Study the drawing (mm; zero at the part's minimum x, y, z) and answer. Coordinates: 2 decimals unless noted, no trailing zeros. Loops run counter-clockwise (first coordinate to the right, second up) from the corner with the lowest first, then second, coordinate; pieces in that order, holes last. Notation, with made-up numbers: (-40, 60) - (-11, 60) arc R14 ccw to (-11, 79) - close; hole circle Ø8 at (20, 61.5). An arc over 180 degrees is marked (long way). One line per item, written item: value. Start each with the question number.
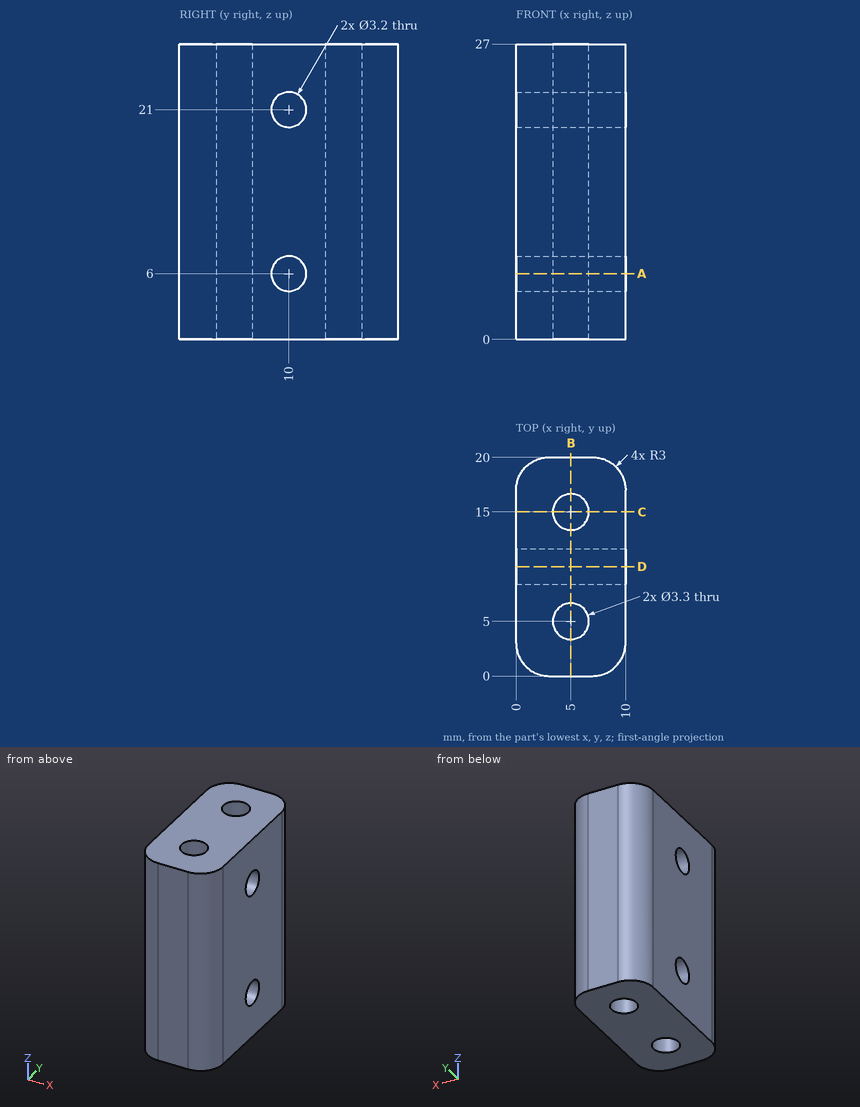
1) Section B-B, the plane x = 5 is taken. Determine the outline of the cut face in (y, z), and give its area (3 significant figures).
2) Section D-D, the plane y = 10 is taken. Determine the outline of the cut face in (x, z).
3) Section C-C, the plane y = 15 is taken. Determine the outline of the cut face in (x, z).
4) Straight lines are drawn through the part: L1, parallel to Y at x = 5, z = 11; L2, parallel to Z at x = 5.5, y = 10; L3, parallel to Y at x = 5, z = 6.25. For each, find the intervals that lie inside material, in ascending order.
5) Section A-A, the plane z = 6 is taken. Determine the outline of the cut face in (x, y).
Answer below:
1. outline: (0, 0) - (3.35, 0) - (3.35, 27) - (0, 27) - close; (6.65, 0) - (13.35, 0) - (13.35, 27) - (6.65, 27) - close; (16.65, 0) - (20, 0) - (20, 27) - (16.65, 27) - close; hole circle Ø3.2 at (10, 6); hole circle Ø3.2 at (10, 21)
1. area: 346 mm2
2. outline: (0, 0) - (10, 0) - (10, 4.4) - (0, 4.4) - close; (0, 7.6) - (10, 7.6) - (10, 19.4) - (0, 19.4) - close; (0, 22.6) - (10, 22.6) - (10, 27) - (0, 27) - close
3. outline: (0, 0) - (3.35, 0) - (3.35, 27) - (0, 27) - close; (6.65, 0) - (10, 0) - (10, 27) - (6.65, 27) - close
4. L1: 0 to 3.35, 6.65 to 13.35, 16.65 to 20
4. L2: 0 to 4.4, 7.6 to 19.4, 22.6 to 27
4. L3: 0 to 3.35, 6.65 to 8.42, 11.58 to 13.35, 16.65 to 20
5. outline: (0, 3) arc R3 ccw to (3, 0) - (7, 0) arc R3 ccw to (10, 3) - (10, 8.4) - (0, 8.4) - close; (0, 11.6) - (10, 11.6) - (10, 17) arc R3 ccw to (7, 20) - (3, 20) arc R3 ccw to (0, 17) - close; hole circle Ø3.3 at (5, 5); hole circle Ø3.3 at (5, 15)
